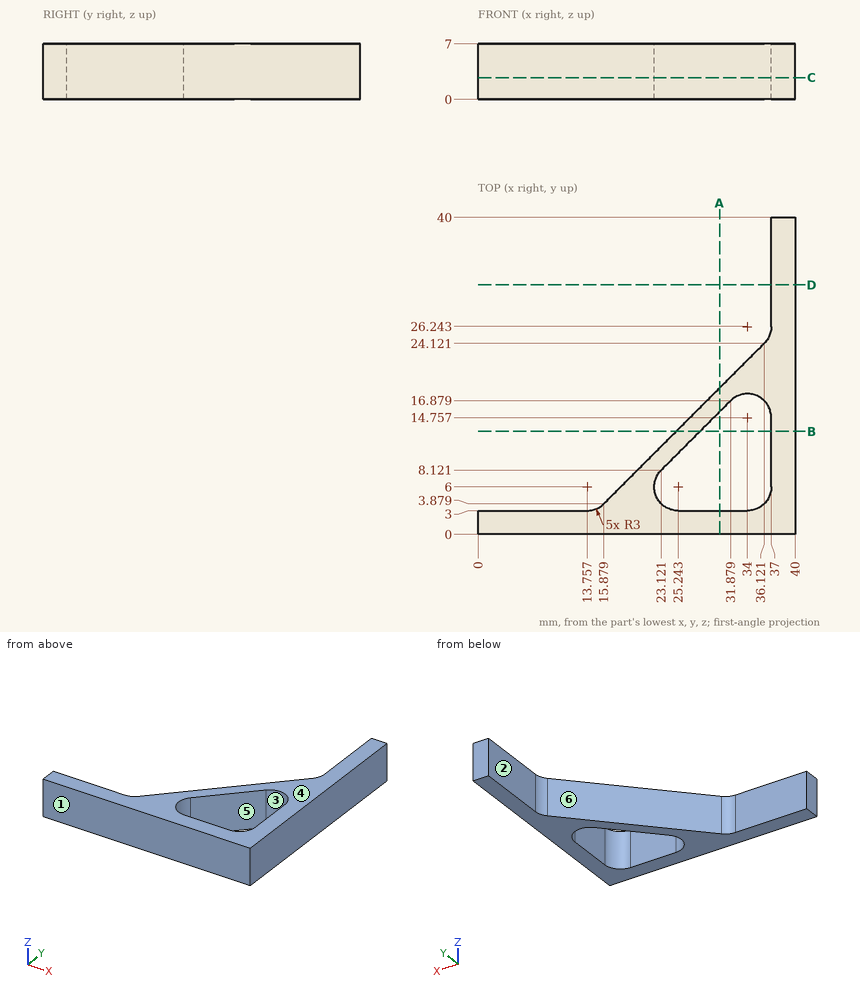
Part print with two shaded views. Sizes in mm from the minimum x, y, z corner. A direction names the side the tool comes from. Coordinates: 2 decimals unless noted, no trailing zeros. Write each loop counter-clockwise with the first axis right and the second up, starting at its lowest first coordinate (ties: lowest second). Pieces come first, ordered by that corner, then holes. Notation, with made-up numbers: (-12.5, -33) - (7.5, -33) arc R29 cw to (7.5, -5) - close; hole circle Ø7 at (5, 48). An arc over 180 degrees is marked (long way). Use a Markdown table: item, result. Add a question column.
Item 1: Two-plate mould, pull along Y, no slides. Class the marked faces 4, 5 and 6: pulls with the +Y half, pulls with the -Y half, needs draft (parallel to the pull), parting line crosses it, or undercut.
Item 2: Band-saw the part on B-B, the plane y = 13. Write the cut outline in (x, z).
Item 3: Drill centre lines: line 1 along X through (y, z) = (31, 0.75); line 2 along Y through (x, z) = (8.5, 3.75); line 3 along Y through (x, z) = (35.5, 1.75) (1 decimal). Where is each one in solid material? Low to high.
Item 4: Band-saw the part on A-A, the plane x = 30.5. Write the cut outline in (y, z), and give its area (3 significant figures).
Item 5: Band-saw the part on D-D, the plane y = 31.5. Write the cut outline in (x, z).
Item 6: Drop flat-ended pins along their axis: pin 1 (2 mm diameter, centred on x = 4.5, z = 3, fed in from +Y); pin 2 (2 mm diameter, centred on x = 27.5, z = 4, fed in from +Y); pin 3 (4 mm diameter, centred on x = 34.5, z = 4.5, fed in from +Y) (1 decimal). Give the stop position or say it passes through.
Item 7: Band-saw the part on C-C, the plane z = 2.75. Write the cut outline in (x, y).
Item 8: 3-axis set-ups, long thin cutter, end or side, ignore diameter. For the marked faces 1, 2 and 3: which of +Z, -Z, +X, -X, +Y, -Y reach the whole face in a straight line?
A:
| question | item | result |
|---|---|---|
| 1 | face 4 | needs draft |
| 1 | face 5 | undercut |
| 1 | face 6 | pulls with the +Y half |
| 2 | outline | (25, 0) - (28, 0) - (28, 7) - (25, 7) - close; (37, 0) - (40, 0) - (40, 7) - (37, 7) - close |
| 3 | line 1 | x = 37 to 40 |
| 3 | line 2 | y = 0 to 3 |
| 3 | line 3 | y = 0 to 3.4, 17.4 to 23.5 |
| 4 | outline | (0, 0) - (3, 0) - (3, 7) - (0, 7) - close; (15.5, 0) - (18.5, 0) - (18.5, 7) - (15.5, 7) - close |
| 4 | area | 42.0 mm² |
| 5 | outline | (37, 0) - (40, 0) - (40, 7) - (37, 7) - close |
| 6 | pin 1 | stops at y = 3 |
| 6 | pin 2 | stops at y = 16.5 |
| 6 | pin 3 | stops at y = 24.6 |
| 7 | outline | (0, 0) - (40, 0) - (40, 40) - (37, 40) - (37, 26.24) arc R3 cw to (36.12, 24.12) - (15.88, 3.88) arc R3 cw to (13.76, 3) - (0, 3) - close; hole (23.12, 8.12) arc R3 ccw to (25.24, 3) - (34, 3) arc R3 ccw to (37, 6) - (37, 14.76) arc R3 ccw to (31.88, 16.88) - close |
| 8 | face 1 | +Z, -Z, +X, -X, -Y |
| 8 | face 2 | +Z, -Z, -X, +Y |
| 8 | face 3 | +Z, -Z |
